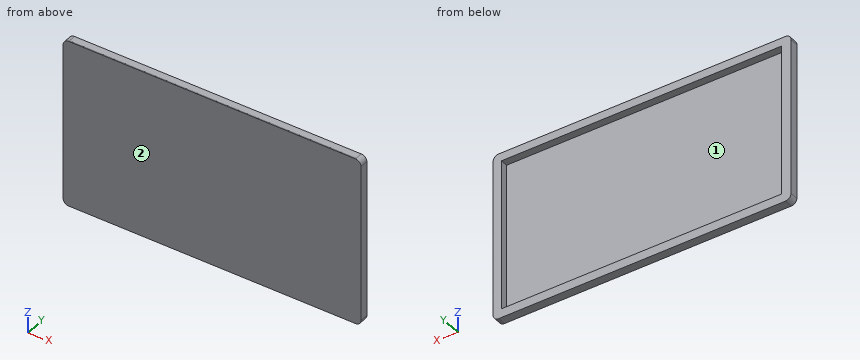
```python
from build123d import *

# Parameters (mm, degrees)
F0_W     = 1600
F0_H     = 900
F0_W_2   = 1504.2692422867
F0_H_2   = 808.7469339371
F1_DEPTH = 40
F2_W     = 1600
F2_H     = 899.8901372014
F3_DEPTH = 5
F4_R     = 30


with BuildPart() as f1:
    # F0 (on Front) → F1 (new body)
    with BuildSketch(Plane.XZ):
        with Locations((30.8563187718, 30.8205480518)):
            Rectangle(F0_W, F0_H)
        with Locations((34.0940356255, 32.6578398405)):
            Rectangle(F0_W_2, F0_H_2, mode=Mode.SUBTRACT)
    extrude(amount=F1_DEPTH)

    # F2 (on face) → F3 (join)
    with BuildSketch(Plane.XZ.offset(40)):
        with Locations((30.8563187718, 30.7656166525)):
            Rectangle(F2_W, F2_H)
    extrude(amount=F3_DEPTH)

    # F4
    f4_edges = [f1.edges().sort_by_distance(p)[0] for p in [
        (830.856319, -22.5, -419.179452),
        (-769.143681, -22.5, -419.179452),
        (-769.143681, -20, 480.820548),
        (830.856319, -20, 480.820548),
    ]]
    fillet(f4_edges, radius=F4_R)


solid = f1.part
```
Verification items for the finished model (mm, model axes). Face numbers are marked on the shaded views. Round coordinates to 2 decimals unless told otherwise and drop trailing zeros. Write each loop counter-clockwise with the first axis right and the second up, starting at its lowest first coordinate (ties: lowest second). Pieces come first, ordered by that corner, then holes. Notation, with made-up numbers: (23, 78.25) - (41, 78.25) arc R26 ccw to (41, 99.25) - close; hole circle Ø10 at (36.25, -28.5). An arc over 180 degrees is marked (long way). Answer as a JSON object with one key per item and string values. Group by question number.
Q1. Section check A-A, the plane y = -7.5. Enter the section's corners in (x, z).
Q2. Thickness scan on line 1 (Z direction, x = 632, y = -25.5); line 2 (X direction, y = -16.5, z = 420.5); line 3 (Y direction, x = -123, z = 207.5). Record the ranges inside material, lowest first.
Q3. Mould release check, pull along X, two halves, no side actions. Record for the marked faces 1 and 2: released by +X, released by -X, zero draft, split by the parting line, or undercut.
Q4. Section check B-B, the plane z = 100.5. Enter the section's corners in (x, y), plus the area to 3 significant figures.
Q5. Go/stop test with flat-tipped pins: pin 1 Ø12 at (x, z) = (374, -143) entering from +Y; pin 2 Ø2.5 at (x, y) = (5.5, -42) entering from +Z. Record where each tip stops, or that it passes through.
Q6. Section check C-C, the plane x = -574.5. Enter the section's corners in (y, z), plus the area to 3 significant figures.
Found:
{
 "1": {"outline": "(-769.14, -389.18) arc R30 ccw to (-739.14, -419.18) - (800.86, -419.18) arc R30 ccw to (830.86, -389.18) - (830.86, 450.82) arc R30 ccw to (800.86, 480.82) - (-739.14, 480.82) arc R30 ccw to (-769.14, 450.82) - close; hole (-718.04, -371.72) - (786.23, -371.72) - (786.23, 437.03) - (-718.04, 437.03) - close"},
 "2": {"line 1": "z = -419.18 to -371.72, 437.03 to 480.82", "line 2": "x = -769.14 to -718.04, 786.23 to 830.86", "line 3": "y = -45 to -40"},
 "3": {"face 1": "undercut", "face 2": "zero draft"},
 "4": {"outline": "(-769.14, -45) - (830.86, -45) - (830.86, 0) - (786.23, 0) - (786.23, -40) - (-718.04, -40) - (-718.04, 0) - (-769.14, 0) - close", "area": "11,800 mm^2"},
 "5": {"pin 1": "stops at y = -40", "pin 2": "stops at z = 480.71"},
 "6": {"outline": "(-45, -419.18) - (0, -419.18) - (0, -371.72) - (-40, -371.72) - (-40, 437.03) - (0, 437.03) - (0, 480.82) - (-40, 480.82) - (-40, 480.71) - (-45, 480.71) - close", "area": "8,150 mm^2"}
}
